```python
from build123d import *

# Parameters (mm, degrees)
F0_W           = 520
F0_H           = 500
F1_DEPTH       = 20
F3_D           = 11
F3_CBORE_D     = 17.25
F3_CBORE_DEPTH = 10
F4_D           = 8
F5_W           = 100
F5_H           = 30
F6_DEPTH       = 20.001


with BuildPart() as f1:
    # F0 (on Top) → F1 (new body)
    with BuildSketch(Plane.XY):
        Rectangle(F0_W, F0_H)
    extrude(amount=F1_DEPTH)

    # F3 (through all)
    with Locations(Plane.XY.offset(20)):
        with Locations((0, 190), (82.4379104323, 171.1840849015), (148.5479816689, 118.4630623532), (185.2363033145, 42.2789774517), (185.2363033145, -42.2789774517), (148.5479816689, -118.4630623532), (82.4379104323, -171.1840849015), (0, -190), (-82.4379104323, -171.1840849015), (-148.5479816689, -118.4630623532), (-185.2363033145, -42.2789774517), (-185.2363033145, 42.2789774517), (-148.5479816689, 118.4630623532), (-82.4379104323, 171.1840849015)):
            CounterBoreHole(F3_D / 2, F3_CBORE_D / 2, F3_CBORE_DEPTH)

    # F4 (through all)
    with Locations(Plane.XY.offset(20)):
        with Locations((0, 0)):
            Hole(F4_D / 2)

    # F5 (on face) → F6 (cut, through all)
    with BuildSketch(Plane.XY.offset(20)):
        with Locations((0, -235)):
            Rectangle(F5_W, F5_H)
    extrude(amount=-F6_DEPTH, mode=Mode.SUBTRACT)


solid = f1.part
```
Model file for the job. Use its own axes, mm. A direction names the side the tool comes from. Give positions to 0.01 mm unless a question says otherwise; leave off trailing zeros.
1) 3-axis set-ups, long thin cutter, end or side, ignore diameter. For faces 5 (the cylindrical face through (79.9, 166.305, 4.93)), 6 (the flat face through (-50, -235, 10)), 7 (the cylindrical face through (-157.165, -118.084, 15.07)): which of +Z, -Z, +X, -X, +Y, -Y reach the whole face in a straight line?
2) Wall check: probe 1 along Y at (x, z) = (148.5, 19); probe 2 along X at (y, z) = (-43, 16.5); probe 3 along X at (y, z) = (-172, 18.5). Give the ranges that are in metal, low to high.
3) Saw through at A-A, the plane z = 3.25. Count the separate pieces of the cut face and the enclosed holes in it, then the cut area to 3 significant figures.
4) Mould opens along Y. For faces 1 (the flat face through (-1, -220, 10)), 2 (the cylindrical face through (-179.74, -42.04, 4.93)), 3 (the flat face through (50, -235, 10)), 4 (the cylindrical face through (81.32, -162.63, 15.07)) say: +Y half, -Y half, draft (parallel to the pull), parting line (faces both ways), or undercut.
5) Pin check, flat tip, straight feed: pin 1 (14 mm diameter, centred on x = 185.24, y = 42.28, fed in from +Z). Stop position of the tip, or through.
Computed:
1. face 5: +Z, -Z
1. face 6: +Z, -Z, -Y
1. face 7: +Z
2. probe 1: y = -250 to -127.09, -109.84 to 109.84, 127.09 to 250
2. probe 2: x = -260 to -193.83, -176.64 to 176.64, 193.83 to 260
2. probe 3: x = -260 to -91.02, -73.85 to 73.85, 91.02 to 260
3. separate pieces: 1
3. enclosed holes: 15
3. area: 256,000 mm2
4. face 1: -Y half
4. face 2: undercut
4. face 3: draft
4. face 4: undercut
5. pin 1: stops at z = 10
